Input: part model. Units: mm. Frame: model coordinates. Face numbers are marked on the shaded views. A direction names the side the tool comes from. Round coordinates to 2 decimals unless told otherwise and drop trailing zeros. Loops run counter-clockwise (first coordinate to the right, second up) from the corner with the lowest first, then second, coordinate; pieces in that order, holes last.
(1) Draft query along Y for the marked faces 1, 2, 3 and 4. Return one class per face: released by +Y, released by -Y, zero draft, split by the parting line, or undercut.
(2) Cut plane B-B, the plane z = -10.25. Output: boundary loops of the cut face in (x, y), and give its area (3 significant figures).
(3) First-contact query: pin 1 Ø1.5 at (y, z) = (27, -4) entering from -X; pin 2 Ø1 at (x, z) = (4, 1.5) entering from -Y; pin 3 Ø1 at (y, z) = (10, 1.5) entering from +X. Flat tips, straight axial feed; report the tip coordinate or a pass-through.
(4) Access query for the marked faces 5 and 6. Directions: +Z, -Z, +X, -X, +Y, -Y. A direction counts if a zero-diameter tool reaches every point of the face in a straight line with its end or side. Return the directions, or none.
(5) Line query: line 1 (X direction, y = 18, z = 0); line 2 (Y direction, x = 0, z = -8.75); line 3 (Z direction, x = 0, y = -0.75). Output: solid intervals per line, ascending.
(6) Cut plane A-A, the plane y = 24.5. Output: boundary loops of the cut face in (x, z).
from build123d import *

# Parameters (mm, degrees)
SKETCH1_R           = 8
BOSS_EXTRUDE1_DEPTH = 30.5
SHELL1_T            = -1.5
SKETCH2_R           = 3.4
BOSS_EXTRUDE2_DEPTH = 5.4
SHELL2_START        = -3.9
SHELL2_OUTLINE_R    = 1.9
SHELL2_DEPTH        = 5.4
SKETCH5_R           = 2.45
BOSS_EXTRUDE5_DEPTH = 4.9
SKETCH6_R           = 1.5
BOSS_EXTRUDE6_DEPTH = 6.3
SKETCH7_R           = 0.95
CUT_EXTRUDE1_DEPTH  = 11.3
SKETCH8_R           = 1.9
CUT_EXTRUDE2_DEPTH  = 39.216750365
FILLET1_R           = 1
FILLET2_R           = 0.5
BOSS_EXTRUDE7_START = -1.5
BOSS_EXTRUDE7_DEPTH = 1.5


# Read off the part's stored shape, not the designer's step: Shell2
with BuildPart() as part:
    # Sketch1 → Boss-Extrude1 (new body)
    with BuildSketch(Plane(origin=(0, 0, 0), x_dir=(1, 0, 0), z_dir=(0, 1, 0))):
        with Locations(Location((0, 0, 0), (0, 0, 90))):
            Circle(SKETCH1_R)
    extrude(amount=BOSS_EXTRUDE1_DEPTH)

    # Shell1
    shell1_openings = [part.faces().sort_by_distance(p)[0] for p in [
        (0, 30.5, 0),
    ]]
    offset(amount=SHELL1_T, openings=shell1_openings, kind=Kind.INTERSECTION)

    # Sketch2 → Boss-Extrude2 (add)
    with BuildSketch(Plane.XZ):
        with Locations(Location((0, -3.4, 0), (0, 0, 90))):
            Circle(SKETCH2_R)
    extrude(amount=BOSS_EXTRUDE2_DEPTH)

    # Shell2 outline → Shell2 (cut)
    with BuildSketch(Plane(origin=(0, 0, 0), x_dir=(1, 0, 0), z_dir=(0, 1, 0)).offset(SHELL2_START)):
        with Locations((0, 3.4)):
            Circle(SHELL2_OUTLINE_R)
    extrude(amount=SHELL2_DEPTH, mode=Mode.SUBTRACT)

    # Sketch5 → Boss-Extrude5 (add)
    with BuildSketch(Plane.XY.offset(-3.4)):
        with Locations((0, -2.35384725)):
            Circle(SKETCH5_R)
    extrude(amount=-BOSS_EXTRUDE5_DEPTH)

    # Sketch6 → Boss-Extrude6 (add)
    with BuildSketch(Plane(origin=(0, 0, -8.3), x_dir=(-1, 0, 0), z_dir=(0, 0, -1))):
        with Locations((0, -2.35384725)):
            Circle(SKETCH6_R)
    extrude(amount=BOSS_EXTRUDE6_DEPTH)

    # Sketch7 → Cut-Extrude1 (cut)
    with BuildSketch(Plane(origin=(0, 0, -14.6), x_dir=(-1, 0, 0), z_dir=(0, 0, -1))):
        with Locations((0, -2.35384725)):
            Circle(SKETCH7_R)
    extrude(amount=-CUT_EXTRUDE1_DEPTH, mode=Mode.SUBTRACT)

    # Sketch8 → Cut-Extrude2 (cut, through all)
    with BuildSketch(Plane(origin=(0, -3.9, 0), x_dir=(1, 0, 0), z_dir=(0, 1, 0))):
        with Locations(Location((0, 3.4, 0), (0, 0, 270))):
            Circle(SKETCH8_R)
    extrude(amount=CUT_EXTRUDE2_DEPTH, mode=Mode.SUBTRACT)

    # Fillet1
    # the kernel refuses this fillet: 1 mm, written as the material it takes off along each edge
    with BuildSketch(Plane(origin=(0, -2.35384725, -14.6), x_dir=(-1, 0, 0), z_dir=(0, -1, 0))) as fillet1_piece_1:
        with BuildLine():
            CenterArc((0.5, -0.893028555), FILLET1_R, 0, 63.25631605)
            Line((1.5, -0.893028555), (1.52, -0.893028555))
            Line((1.52, -0.893028555), (1.52, 0))
            Line((1.52, 0), (1.5, 0.02))
            ThreePointArc((1.5, 0.02), (1.225, 0.02), (0.959, 0.017860571))
            Line((0.959, 0.017860571), (0.95, 0))
        make_face()
    revolve(axis=Axis((0, -2.35384725, -14.6), (0, 0, -1)), mode=Mode.SUBTRACT)

    # Fillet2
    fillet2_edges = [part.edges().sort_by_distance(p)[0] for p in [
        (0, 30.5, 8),
    ]]
    fillet(fillet2_edges, radius=FILLET2_R)

    # Sketch9 → Boss-Extrude7 (add)
    with BuildSketch(Plane(origin=(0, 30.5, 0), x_dir=(1, 0, 0), z_dir=(0, 1, 0)).offset(BOSS_EXTRUDE7_START)):
        with BuildLine():
            Line((-10.637668918, 2.8), (-5.86600375, 2.8))
            ThreePointArc((-5.86600375, 2.8), (-6.5, 0), (-5.86600375, -2.8))
            Line((-5.86600375, -2.8), (-10.637668918, -2.8))
            ThreePointArc((-10.637668918, -2.8), (-11, 0), (-10.637668918, 2.8))
        make_face()
    extrude(amount=BOSS_EXTRUDE7_DEPTH)

    # Mirror1: part across plane


with BuildPart() as part_1:
    add(part.part)
    add(part.part.mirror(Plane(origin=(0, 0, 0), x_dir=(0, 0, 1), z_dir=(1, 0, 0))))


solid = part_1.part
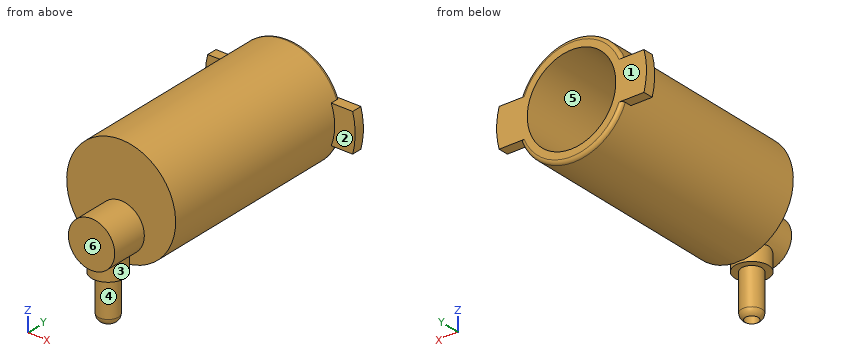
Reported:
1. face 1: released by +Y
1. face 2: released by -Y
1. face 3: undercut
1. face 4: split by the parting line
2. outline: circle Ø3 at (0, -2.35); hole circle Ø1.9 at (0, -2.35)
2. area: 4.23 mm2
3. pin 1: stops at x = -7.31
3. pin 2: stops at y = 0
3. pin 3: stops at x = 7.94
4. face 5: +Y
4. face 6: +Z, -Z, +X, -X, -Y
5. line 1: x = -8 to -6.5, 6.5 to 8
5. line 2: y = -3.85 to -3.3, -1.4 to -0.85
5. line 3: z = -8.3 to -5.3, -1.5 to 0
6. outline: circle Ø16 at (0, 0); hole circle Ø13 at (0, 0)
